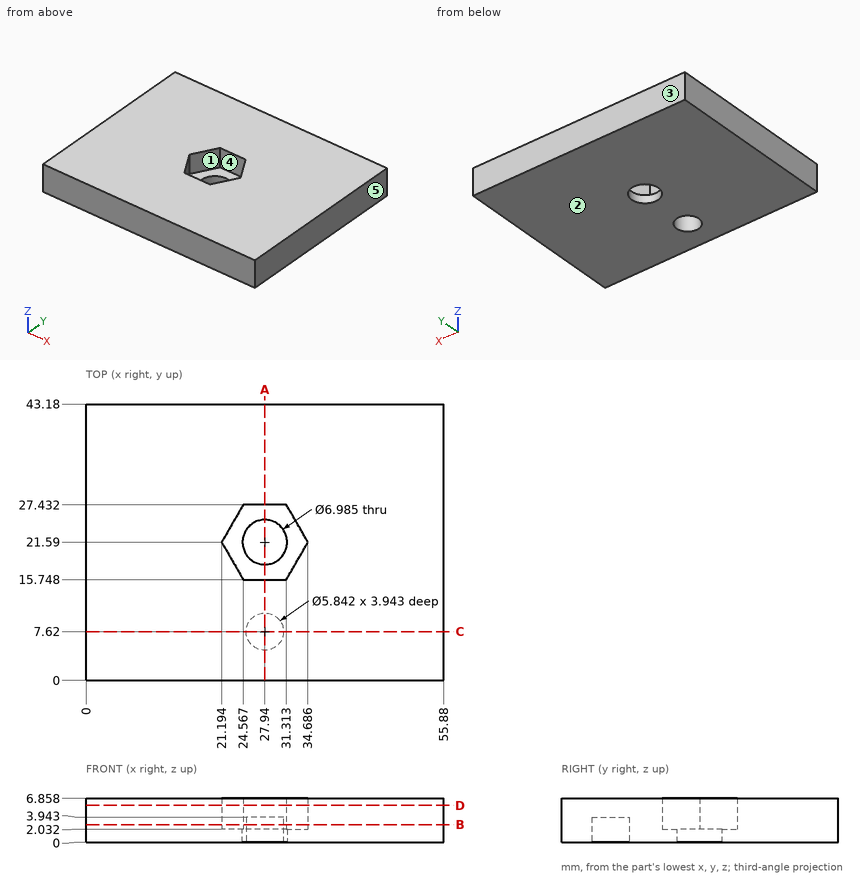
Answer from the drawing. Dimensions are ordinates in mm from the lowest x, y and z of the part. A direction names the side the tool comes from. Give positions to 0.01 mm unless a question says otherwise; leave off trailing zeros. Order: outer loops, then holes, each group sorted by start corner. A loop starts at its lowest first (then second) coordinate and runs counter-clockwise, first axis right, second up. Notation, with made-up numbers: (31, 78) - (63, 78) arc R34 ccw to (63, 114) - close; hole circle Ø9 at (36.25, 80.25). An arc over 180 degrees is marked (long way). One line per item, written item: value. Start each with the question number.
1) Given pin 1 Ø4 at (x, y) = (30.5, 19) entering from +Z; pin 2 Ø1.5 at (x, y) = (29.5, 35) entering from -Z; pin 3 Ø4 at (x, y) = (27.94, 21.59) entering from +Z, each flat-ended and moving along its own axis, determine where each tip first touches the part or whether it passes through.
2) A cutting plane is placed at B-B on z = 2.75. Give the vertices of the cut face in (x, y).
3) A cutting plane is placed at D-D on z = 5.75. Give the vertices of the cut face in (x, y), then the cut area to 3 significant figures.
4) A tool of negligible diameter and unlimited length cuts with its end or side. For the marked faces 1 and 2, from which of +Z, -Z, +X, -X, +Y, -Y can it reach the whole face along a straight path? Write none if from no direction.
5) A cutting plane is placed at A-A on x = 27.94. Give the vertices of the cut face in (y, z).
6) The mould has two halves that part along Y. Classify the marked faces 3, 4 and 5: released by +Y, released by -Y, zero draft, split by the parting line, or undercut.
7) Find the intervals of material crossed by L1, parallel to Y at x = 27.94, z = 0.65; L2, parallel to Y at x = 27.94, z = 2.95; L3, parallel to X at y = 7.62, z = 3.1, in increasing order.
8) A cutting plane is placed at C-C on y = 7.62. Give the vertices of the cut face in (x, z).
Answer sheet:
1. pin 1: stops at z = 2.03
1. pin 2: stops at z = 0
1. pin 3: passes through
2. outline: (0, 0) - (55.88, 0) - (55.88, 43.18) - (0, 43.18) - close; hole (21.19, 21.59) - (24.57, 15.75) - (31.31, 15.75) - (34.69, 21.59) - (31.31, 27.43) - (24.57, 27.43) - close; hole circle Ø5.84 at (27.94, 7.62)
3. outline: (0, 0) - (55.88, 0) - (55.88, 43.18) - (0, 43.18) - close; hole (21.19, 21.59) - (24.57, 15.75) - (31.31, 15.75) - (34.69, 21.59) - (31.31, 27.43) - (24.57, 27.43) - close
3. area: 2,290 mm2
4. face 1: +Z
4. face 2: -Z, +X, -X, +Y, -Y
5. outline: (0, 0) - (4.7, 0) - (4.7, 3.94) - (10.54, 3.94) - (10.54, 0) - (18.1, 0) - (18.1, 2.03) - (15.75, 2.03) - (15.75, 6.86) - (0, 6.86) - close; (25.08, 0) - (43.18, 0) - (43.18, 6.86) - (27.43, 6.86) - (27.43, 2.03) - (25.08, 2.03) - close
6. face 3: released by +Y
6. face 4: undercut
6. face 5: zero draft
7. L1: y = 0 to 4.7, 10.54 to 18.1, 25.08 to 43.18
7. L2: y = 0 to 4.7, 10.54 to 15.75, 27.43 to 43.18
7. L3: x = 0 to 25.02, 30.86 to 55.88
8. outline: (0, 0) - (25.02, 0) - (25.02, 3.94) - (30.86, 3.94) - (30.86, 0) - (55.88, 0) - (55.88, 6.86) - (0, 6.86) - close
